Drawing for the job (mm, zero at the part's lowest x, y, z). A direction names the side the tool comes from. Round coordinates to 2 decimals unless told otherwise and drop trailing zeros. Loops run counter-clockwise (first coordinate to the right, second up) from the corner with the lowest first, then second, coordinate; pieces in that order, holes last. Notation, with made-up numbers: M 26,21.25 L 52,21.25 A27 cw 52,52.25 Z; hole C -19,50 d10. An arc over 180 degrees is marked long. Answer in a Markdown table with one row per item.
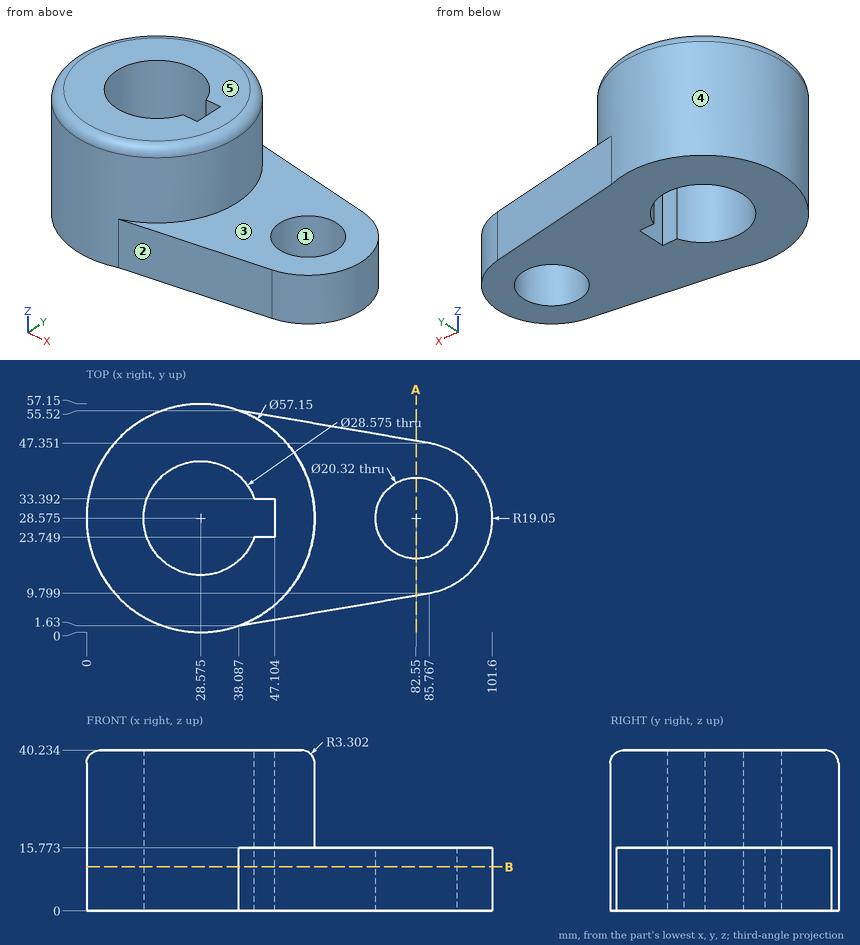
1. Mould opens along Y. For the marked faces 1, 2 and 3 say: +Y half, -Y half, draft (parallel to the pull), parting line (faces both ways), or undercut.
Verdict:
| item | result |
|---|---|
| face 1 | undercut |
| face 2 | -Y half |
| face 3 | draft |
2. Wall check: probe 1 along X at (y, z) = (27.5, 2) (1 decimal); probe 2 along X at (y, z) = (35, 5.5) (1 decimal); probe 3 along Z at (x, y) = (63, 25). Give the ranges that are in metal, low to high.
Verdict:
| item | result |
|---|---|
| probe 1 | x = 0 to 14.3, 47.1 to 72.4, 92.7 to 101.6 |
| probe 2 | x = 0.7 to 15.8, 41.3 to 74.7, 90.4 to 100.5 |
| probe 3 | z = 0 to 15.77 |
3. Pin check, flat tips, straight feed: pin 1 (5 mm diameter, centred on x = 10.5, z = 7, fed in from +Y); pin 2 (2.5 mm diameter, centred on x = 44, z = 20, fed in from +Y); pin 3 (16 mm diameter, centred on x = 72.5, y = 16, fed in from +Z). Stop position of each tip, or through.
Verdict:
| item | result |
|---|---|
| pin 1 | stops at y = 52.53 |
| pin 2 | stops at y = 53.39 |
| pin 3 | stops at z = 15.77 |
4. Tool access for the marked faces 4 and 5: list every direction of +Z, -Z, +X, -X, +Y, -Y with a clear straight run to the whole face (end or side of a thin tool).
Verdict:
| item | result |
|---|---|
| face 4 | +Z |
| face 5 | +Z, +X, -X, +Y, -Y |
5. Saw through at A-A (x = 82.55). Write the cut outline in (y, z) (1 decimal), and give its area (3 significant figures).
Verdict:
| item | result |
|---|---|
| outline | M 9.2,0 L 18.4,0 L 18.4,15.8 L 9.2,15.8 Z; M 38.7,0 L 47.9,0 L 47.9,15.8 L 38.7,15.8 Z |
| area | 289 mm² |
6. Saw through at B-B (z = 11). State how many separate pieces and enclosed holes the cut face has, and give its area (4 significant figures).
Verdict:
| item | result |
|---|---|
| separate pieces | 1 |
| enclosed holes | 2 |
| area | 3,435 mm² |
